Source: three-view drawing plus pictorial views. Frame: mm from the lowest corner of the part. A direction names the side the tool comes from. Coordinates: 2 decimals unless noted, no trailing zeros. Loops run counter-clockwise (first coordinate to the right, second up) from the corner with the lowest first, then second, coordinate; pieces in that order, holes last.
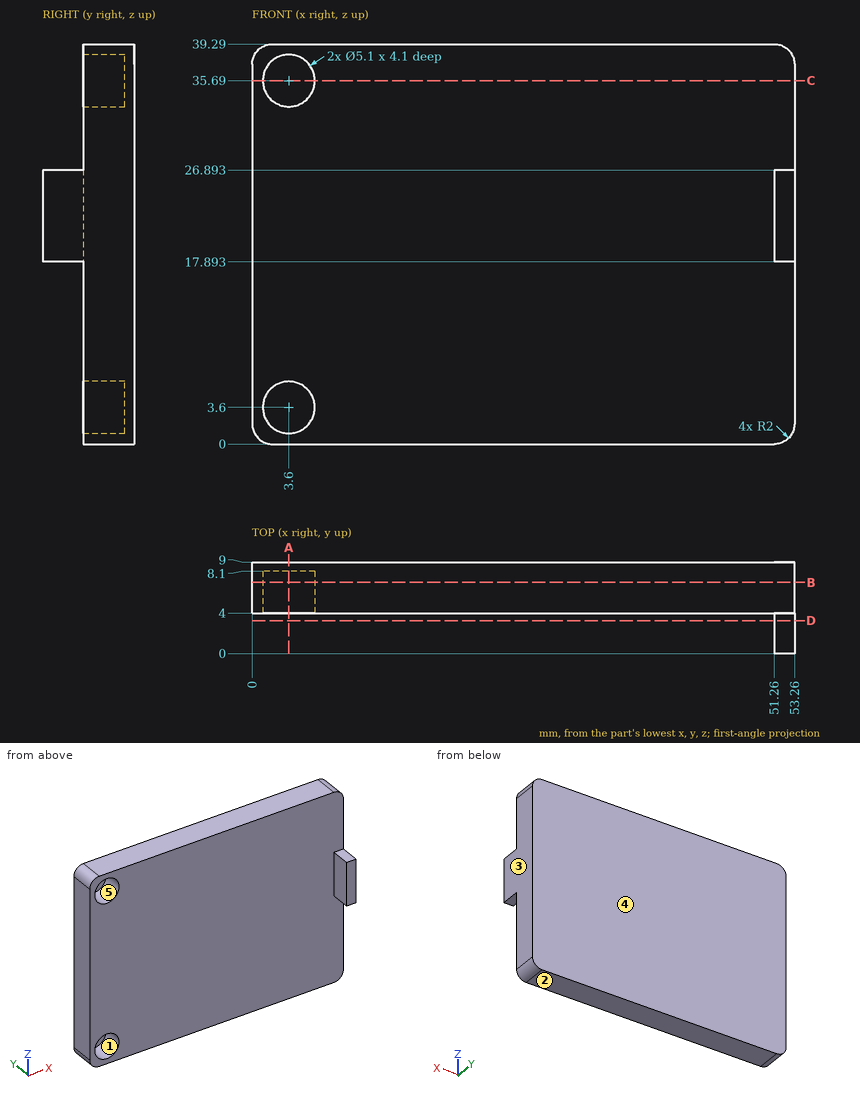
Q1. Section B-B, the plane y = 7. Return the cut outline in (x, z).
Q2. Contact query for flat-ended pins moving along their axis: pin 1 Ø3 at (x, z) = (3.6, 3.6) entering from -Y; pin 2 Ø0.6 at (x, y) = (52.5, 2.5) entering from +Z; pin 3 Ø3 at (x, y) = (39, 1) entering from -Z; pin 4 Ø4 at (x, z) = (3, 3.5) entering from -Y. Output: stop coordinate, or through.
Q3. Access query for the marked faces 1 and 2. Directions: +Z, -Z, +X, -X, +Y, -Y. A direction counts if a zero-diameter tool reaches every point of the face in a straight line with its end or side. Return the directions, or none.
Q4. Section D-D, the plane y = 3.25. Return the cut outline in (x, z).
Q5. Section A-A, the plane x = 3.6. Return the cut outline in (y, z).
Q6. Draft query along X for the marked faces 3, 4 and 5. Return one class per face: +X half, -X half, draft (parallel to the pull), parting line (faces both ways), or undercut.
Q7. Section C-C, the plane z = 35.69. Return the cut outline in (x, y), plus the area to 3 significant figures.
Q8. Line query: line 1 along X through (y, z) = (6.8, 35.69); line 2 along Y through (x, z) = (18, 28); line 3 along X through (y, z) = (2.75, 20). Output: solid intervals per line, ascending.
Derived:
1. outline: (0, 2) arc R2 ccw to (2, 0) - (51.26, 0) arc R2 ccw to (53.26, 2) - (53.26, 37.29) arc R2 ccw to (51.26, 39.29) - (2, 39.29) arc R2 ccw to (0, 37.29) - close; hole circle Ø5.1 at (3.6, 3.6); hole circle Ø5.1 at (3.6, 35.69)
2. pin 1: stops at y = 8.1
2. pin 2: stops at z = 26.89
2. pin 3: passes through
2. pin 4: stops at y = 4
3. face 1: -Y
3. face 2: -Z, +X, -X, +Y, -Y
4. outline: (51.26, 17.89) - (53.26, 17.89) - (53.26, 26.89) - (51.26, 26.89) - close
5. outline: (4, 0) - (9, 0) - (9, 39.29) - (4, 39.29) - (4, 38.24) - (8.1, 38.24) - (8.1, 33.14) - (4, 33.14) - (4, 6.15) - (8.1, 6.15) - (8.1, 1.05) - (4, 1.05) - close
6. face 3: +X half
6. face 4: draft
6. face 5: undercut
7. outline: (0, 4) - (1.05, 4) - (1.05, 8.1) - (6.15, 8.1) - (6.15, 4) - (53.26, 4) - (53.26, 9) - (0, 9) - close
7. area: 245 mm2
8. line 1: x = 0 to 1.05, 6.15 to 53.26
8. line 2: y = 4 to 9
8. line 3: x = 51.26 to 53.26
